Design review of the part built by this model. Coordinates are the model's own, in mm. A direction names the side the tool comes from. Give positions to 0.01 mm unless a question says otherwise; leave off trailing zeros. Loops run counter-clockwise (first coordinate to the right, second up) from the corner with the lowest first, then second, coordinate; pieces in that order, holes last. Notation, with made-up numbers: (32, 57.5) - (85, 57.5) arc R23 ccw to (85, 85.5) - close; hole circle Ø2 at (-29.5, -18). An arc over 180 degrees is marked (long way). Put each result on its own line as item: value. Start each with the question number.
Autodesk Inventor part; units mm, degrees
ref_plane "YZ Plane" through (0, 0, 0) normal (1, 0, 0) x (0, 1, 0)
ref_plane "XZ Plane" through (0, 0, 0) normal (0, 1, 0) x (-1, 0, 0)
ref_plane "XY Plane" through (0, 0, 0) normal (0, 0, 1) x (1, 0, 0)
sketch "Sketch1" plane through (0, 0, 0) normal (0, 1, 0) x (-1, 0, 0)
  line L0 (0, 0) -> (-25.4, 0)
  line L1 (0, 0) -> (0, -25.4)
  line L2 (-1.5875, -25.4) -> (-1.5875, -1.5875)
  line L3 (-1.5875, -1.5875) -> (-25.4, -1.5875)
  line L4 (0, -25.4) -> (-1.5875, -25.4)
  line L5 (-25.4, -1.5875) -> (-25.4, 0)
  dimension "d5" = 25.4
  dimension "d6" = 25.4
  dimension "d7" = 1.5875
extrude "Extrusion1" add sketch "Sketch1" along normal blind 508
sketch "Sketch2" plane through (25.4, 0, -1.5875) normal (0, 0, -1) x (-1, 0, 0)
  line L0 (0, 508) -> (23.8125, 508)
  line L1 (25.4, 0) -> (0, 0)
  line L2 (0, 0) -> (0, 508)
  point P0 (12.7, 425.45)
  point P1 (12.7, 82.55)
  dimension "d10" = 82.55
  dimension "d11" = 82.55
  dimension "d12" = 12.7
  dimension "d13" = 12.7
hole "Hole1" at (12.7, 425.45, -1.5875) at (12.7, 82.55, -1.5875) direction (0, 0, 1) diameter 6.35 end through all
properties part number "gripper main bracket"
Item 1: Consider section B-B (z = -16.5). State the section outline as (x, y) points, plus the area to 3 significant figures.
Item 2: Consider section A-A (y = 135.5). State the section outline as (x, z) points, plus the area to 3 significant figures.
Item 3: Machinability: for faces 4 (the flat face through (1.588, 250, -14)), 5 (the flat face through (7, 0, -1)), which of the approach directions +Z, -Z, +X, -X, +Y, -Y give a long, thin tool a straight path to every point of the face, cutting with its end or side? Answer none if there is none.
Item 4: For P1, Ø10, axis at x = 13, z = -11, coming from the -Y side; P2, Ø12, axis at x = 13, y = 376.5, coming from the -Z side; P3, Ø4, axis at y = 55.5, z = -7, coming from the +X side, all flat-tipped, find the tip position at first contact; note any pin that passes through.
Item 5: Mouldability with a two-part tool opening along Z and no side actions: class faces 1 (the flat face through (13, 250, 0)), 2 (the flat face through (13, 250, -1.588)), 3 (the flat face through (7, 508, -1)) as pulls with the +Z half, pulls with the -Z half, needs draft (parallel to the pull), parting line crosses it, or undercut.
Item 6: For L1, parallel to Y at x = 12.7, z = -0.65 (3 decimals); L2, parallel to X at y = 425.45, z = -0.5 (3 decimals); L3, parallel to X at y = 248, z = -2.25, list the stretches that pass through material, from the lowest coordinate up. Write a range as from..to.
Geometry says:
1. outline: (0, 0) - (1.59, 0) - (1.59, 508) - (0, 508) - close
1. area: 806 mm2
2. outline: (0, -25.4) - (1.59, -25.4) - (1.59, -1.59) - (25.4, -1.59) - (25.4, 0) - (0, 0) - close
2. area: 78.1 mm2
3. face 4: -Z, +X, +Y, -Y
3. face 5: +Z, -Z, +X, -X, -Y
4. P1: passes through
4. P2: stops at z = -1.59
4. P3: stops at x = 1.59
5. face 1: pulls with the +Z half
5. face 2: pulls with the -Z half
5. face 3: needs draft
6. L1: y = 0..79.375, 85.725..422.275, 428.625..508
6. L2: x = 0..9.525, 15.875..25.4
6. L3: x = 0..1.59
